Can you work these out from the drawing? Everything is in mm from the part's minimum corner. Give positions to 0.01 mm unless a question says otherwise; leave off trailing zeros. Order: outer loops, then holes, each group sorted by start corner. A loop starts at its lowest first (then second) coordinate and runs counter-clockwise, first axis right, second up. Notation, with made-up numbers: (35.25, -7) - (89.25, -7) arc R34 cw to (89.25, 31) - close; hole circle Ø5 at (-36.75, -16.75). An arc over 180 degrees is marked (long way). Answer as a JSON object with one key per item and string values.
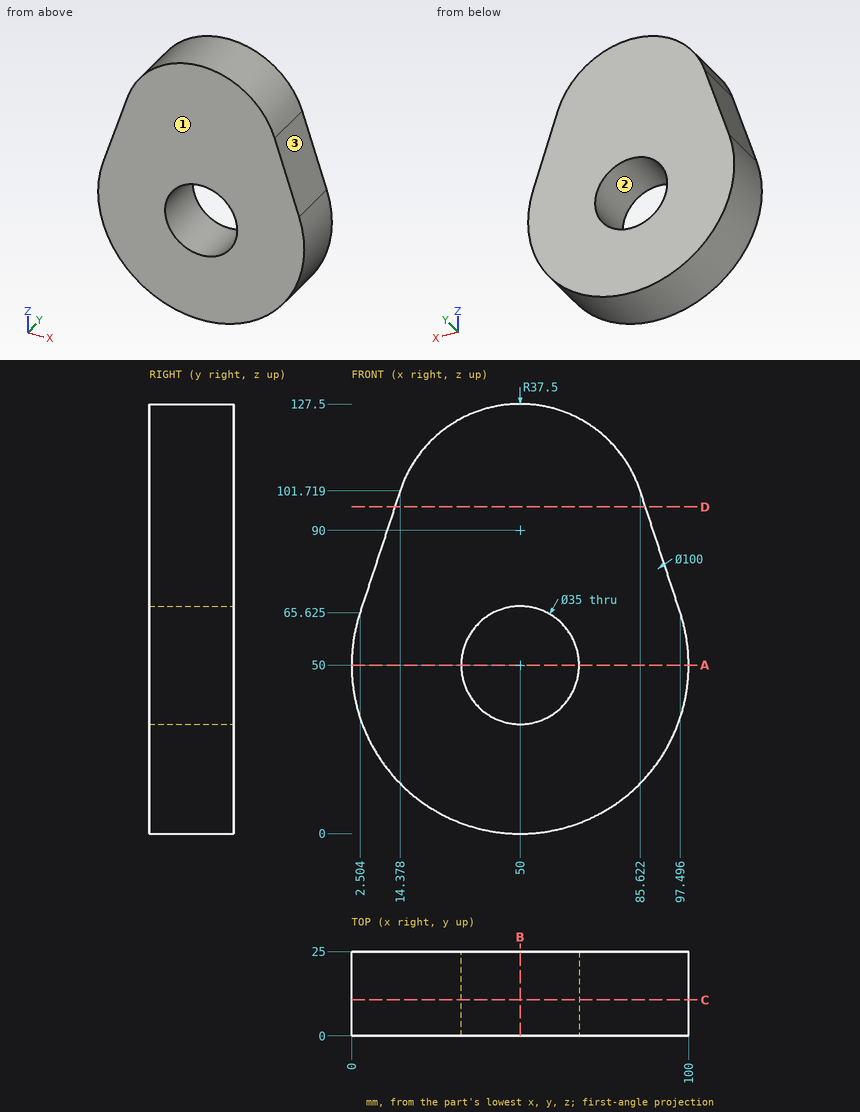
Q1. If we section it at D-D, the plane z = 97: Please give me the cut outline in (x, y), then the cut area to 3 significant figures.
Recorded:
{"outline": "(12.83, 0) - (87.17, 0) - (87.17, 25) - (12.83, 25) - close", "area": "1,860 mm^2"}
Q2. I'm going to push flat-ended pins straight in: pin 1 Ø6 at (y, z) = (10.5, 73.5) entering from +X; pin 2 Ø4 at (x, z) = (35.5, 59.5) entering from -Y; pin 3 Ø1.5 at (y, z) = (13, 46.5) entering from +X; pin 4 Ø4 at (y, z) = (6, 69) entering from -X. Where does each tip first touch, or does it pass through?
Recorded:
{"pin 1": "stops at x = 95.89", "pin 2": "stops at y = 0", "pin 3": "stops at x = 99.92", "pin 4": "stops at x = 2.96"}
Q3. We'd pull the mould along Z, two halves only. Please class the marked faces 1, 2 and 3: released by +Z, released by -Z, zero draft, split by the parting line, or undercut.
Recorded:
{"face 1": "zero draft", "face 2": "undercut", "face 3": "released by +Z"}
Q4. If we section it at C-C, the plane y = 10.75: Please give me the cut outline in (x, z) (1 decimal).
Recorded:
{"outline": "(2.5, 65.6) arc R50 ccw (long way) to (97.5, 65.6) - (85.6, 101.7) arc R37.5 ccw to (14.4, 101.7) - close; hole circle Ø35 at (50, 50)"}
Q5. If we section it at B-B, the plane x = 50: Please give me the cut outline in (y, z).
Recorded:
{"outline": "(0, 0) - (25, 0) - (25, 32.5) - (0, 32.5) - close; (0, 67.5) - (25, 67.5) - (25, 127.5) - (0, 127.5) - close"}
Q6. I need wall thicknesses on L1, parallel to Z at x = 49.5, y = 9.25; L2, parallel to X at y = 17.75, z = 34; L3, parallel to X at y = 11.5, z = 60. Which ranges of each line are inside material? Lowest first, please.
Recorded:
{"L1": "z = 0 to 32.51, 67.49 to 127.5", "L2": "x = 2.63 to 42.91, 57.09 to 97.37", "L3": "x = 1.01 to 35.64, 64.36 to 98.99"}
Q7. If we section it at A-A, the plane z = 50: Please give me the cut outline in (x, y), then the cut area to 4 significant figures.
Recorded:
{"outline": "(0, 0) - (32.5, 0) - (32.5, 25) - (0, 25) - close; (67.5, 0) - (100, 0) - (100, 25) - (67.5, 25) - close", "area": "1,625 mm^2"}
